```python
from build123d import *

# Parameters (mm, degrees)
SKETCH_1_W      = 6.5
SKETCH_1_H      = 3.4
EXTRUDE_1_DEPTH = 5
FILLET_1_R      = 1
CHAMFER_1_SIZE  = 0.5
SKETCH_2_W      = 7
SKETCH_2_H      = 4
EXTRUDE_2_DEPTH = 1
FILLET_2_R      = 0.8


with BuildPart() as part:
    # 草图1 → 凸台-拉伸1 (new body)
    with BuildSketch(Plane.XY):
        Rectangle(SKETCH_1_W, SKETCH_1_H)
    extrude(amount=EXTRUDE_1_DEPTH)

    # 圆角1
    fillet_1_edges = [part.edges().sort_by_distance(p)[0] for p in [
        (3.25, -1.7, 2.5),
        (-3.25, -1.7, 2.5),
        (-3.25, 1.7, 2.5),
        (3.25, 1.7, 2.5),
    ]]
    fillet(fillet_1_edges, radius=FILLET_1_R)

    # 倒角1
    chamfer_1_edges = [part.edges().sort_by_distance(p)[0] for p in [
        (-3.25, 0, 5),
        (0, 1.7, 5),
        (3.25, 0, 5),
        (0, -1.7, 5),
        (-2.957106781, -1.407106781, 5),
        (2.957106781, -1.407106781, 5),
        (2.957106781, 1.407106781, 5),
        (-2.957106781, 1.407106781, 5),
    ]]
    chamfer(chamfer_1_edges, length=CHAMFER_1_SIZE)

    # 草图2 → 凸台-拉伸2 (add)
    with BuildSketch(Plane(origin=(0, 0, 0), x_dir=(-1, 0, 0), z_dir=(0, 0, -1))):
        Rectangle(SKETCH_2_W, SKETCH_2_H)
    extrude(amount=EXTRUDE_2_DEPTH)

    # 圆角2
    fillet_2_edges = [part.edges().sort_by_distance(p)[0] for p in [
        (3.5, 2, -0.5),
        (3.5, -2, -0.5),
        (-3.5, -2, -0.5),
        (-3.5, 2, -0.5),
    ]]
    fillet(fillet_2_edges, radius=FILLET_2_R)


solid = part.part
```
CAD build for the part. Positions are in the model's coordinates, mm. A direction names the side the tool comes from. Round coordinates to 2 decimals unless told otherwise and drop trailing zeros. Loops run counter-clockwise (first coordinate to the right, second up) from the corner with the lowest first, then second, coordinate; pieces in that order, holes last. Notation, with made-up numbers: M 31.5,54.5 L 70.5,54.5 A13 ccw 70.5,67.5 Z; hole C 21,84.5 d10. An arc over 180 degrees is marked long. Use a Markdown table: item, result. Add a question column.
(1) Flat gauge pins, fed straight in: pin 1 (1.1 mm diameter, centred on y = 0, z = 2.5, fed in from -X); pin 2 (2 mm diameter, centred on x = -0.5, z = 3, fed in from -Y); pin 3 (1.5 mm diameter, centred on y = 0, z = 2.5, fed in from +X). Where does each tip first touch, or does it go through?
(2) Which spindle directions (+Z, -Z, +X, -X, +Y, -Y) get a long thin tool onto all of the face, cutting with end or side? Do faces 1 (the face through (0, -1.7, 2)), 2 (the face through (-3.25, 0, 2)), 3 (the face through (-2.965, -1.399, 2.282)), 4 (the face through (2.965, 1.399, 2.282)), 5 (the face through (3.25, 0, 2)). Say none if no direction does.
(3) Cut at D-D (z = 1.95). Give the cut face in (x, y), and give its area (3 significant figures).
(4) Cut at A-A (x = -0.5). Give the cut face in (y, z), and give its area (4 significant figures).
(5) Cut at B-B (y = 0.15). Give the cut face in (x, z).
(6) Drill centre lines: line 1 (Y direction, x = -0.25, z = 3.95); line 2 (Z direction, x = 3.25, y = -1); line 3 (X direction, y = 0, z = 3.8). Where is each one in solid material? Low to high.
(7) Cut at C-C (z = -0.6). Give the cut face in (x, y), and give its area (3 significant figures).
Geometry says:
| question | item | result |
|---|---|---|
| 1 | pin 1 | stops at x = -3.25 |
| 1 | pin 2 | stops at y = -1.7 |
| 1 | pin 3 | stops at x = 3.25 |
| 2 | face 1 | +Z, +X, -X, -Y |
| 2 | face 2 | +Z, -X, +Y, -Y |
| 2 | face 3 | +Z, -X, -Y |
| 2 | face 4 | +Z, +X, +Y |
| 2 | face 5 | +Z, +X, +Y, -Y |
| 3 | outline | M -3.25,-0.7 A1 ccw -2.25,-1.7 L 2.25,-1.7 A1 ccw 3.25,-0.7 L 3.25,0.7 A1 ccw 2.25,1.7 L -2.25,1.7 A1 ccw -3.25,0.7 Z |
| 3 | area | 21.2 mm² |
| 4 | outline | M -2,-1 L 2,-1 L 2,0 L 1.7,0 L 1.7,4.5 L 1.2,5 L -1.2,5 L -1.7,4.5 L -1.7,0 L -2,0 Z |
| 4 | area | 20.75 mm² |
| 5 | outline | M -3.5,-1 L 3.5,-1 L 3.5,0 L 3.25,0 L 3.25,4.5 L 2.75,5 L -2.75,5 L -3.25,4.5 L -3.25,0 L -3.5,0 Z |
| 6 | line 1 | y = -1.7 to 1.7 |
| 6 | line 2 | z = -1 to 0 |
| 6 | line 3 | x = -3.25 to 3.25 |
| 7 | outline | M -3.5,-1.2 A0.8 ccw -2.7,-2 L 2.7,-2 A0.8 ccw 3.5,-1.2 L 3.5,1.2 A0.8 ccw 2.7,2 L -2.7,2 A0.8 ccw -3.5,1.2 Z |
| 7 | area | 27.5 mm² |
